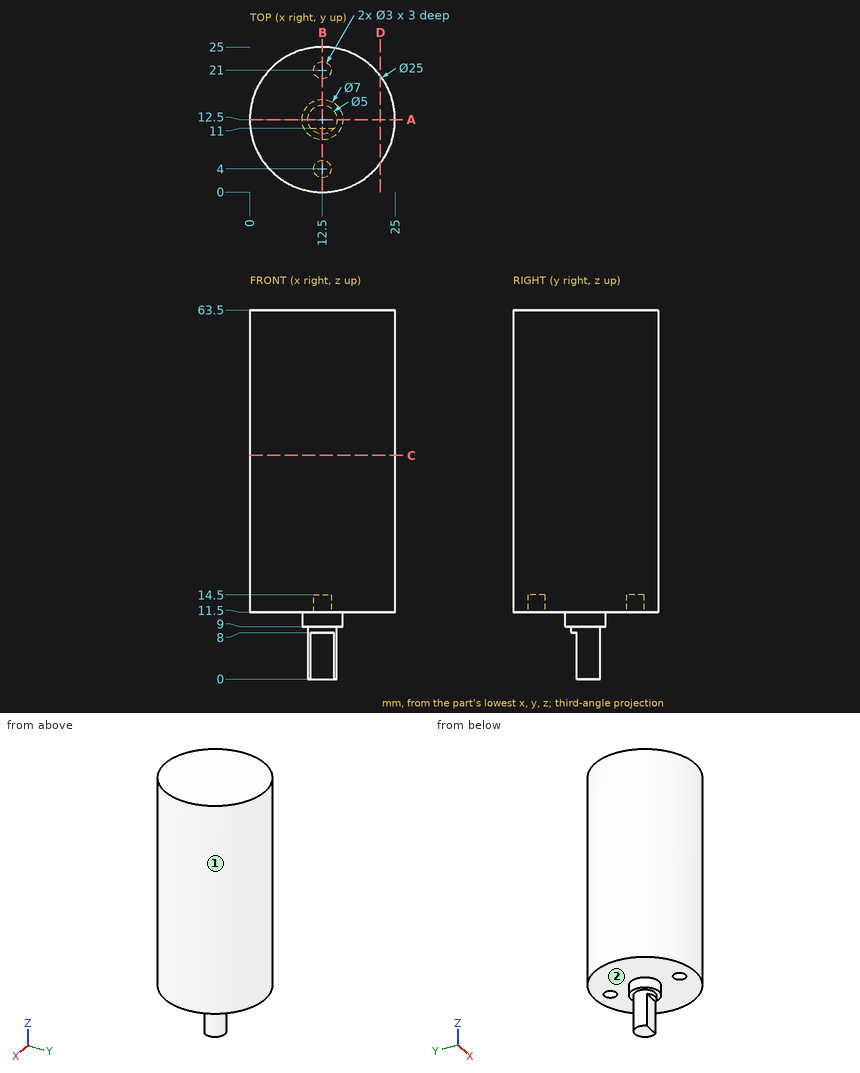
Drawing for the job (mm, zero at the part's lowest x, y, z). A direction names the side the tool comes from. Round coordinates to 2 decimals unless told otherwise and drop trailing zeros. Loops run counter-clockwise (first coordinate to the right, second up) from the corner with the lowest first, then second, coordinate; pieces in that order, holes last.
1. Drop flat-ended pins along their axis: P1, Ø12, axis at x = 4.5, z = 7.5, coming from the +Y side; P2, Ø6, axis at x = 8.5, z = 52.5, coming from the +Y side; P3, Ø6, axis at x = 19.5, z = 43.5, coming from the -Y side; P4, Ø5.5, axis at x = 11, y = 11.5, coming from the -Z side. Give the stop position or say it passes through.
Check values:
P1: stops at y = 24.49
P2: stops at y = 24.96
P3: stops at y = 0.66
P4: stops at z = 0
2. Band-saw the part on A-A, the plane y = 12.5. List the corners of the cut face in (x, z), and give its area (3 significant figures).
Check values:
outline: (0, 11.5) - (9, 11.5) - (9, 9) - (10, 9) - (10, 0) - (15, 0) - (15, 9) - (16, 9) - (16, 11.5) - (25, 11.5) - (25, 63.5) - (0, 63.5) - close
area: 1,360 mm2
3. Tool access for the marked faces 1 and 2: list every direction of +Z, -Z, +X, -X, +Y, -Y with a clear straight run to the whole face (end or side of a thin tool).
Check values:
face 1: +Z, -Z
face 2: -Z
4. Wall check: probe 1 along Y at (x, z) = (12.5, 12.55); probe 2 along Z at (x, y) = (19, 12.25); probe 3 along Y at (x, z) = (13, 54). Give the ranges that are in metal, low to high.
Check values:
probe 1: y = 0 to 2.5, 5.5 to 19.5, 22.5 to 25
probe 2: z = 11.5 to 63.5
probe 3: y = 0.01 to 24.99
5. Band-saw the part on B-B, the plane x = 12.5. List the corners of the cut face in (y, z), and give its area (3 significant figures).
Check values:
outline: (0, 11.5) - (2.5, 11.5) - (2.5, 14.5) - (5.5, 14.5) - (5.5, 11.5) - (9, 11.5) - (9, 9) - (10, 9) - (10, 8) - (11, 8) - (11, 0) - (15, 0) - (15, 9) - (16, 9) - (16, 11.5) - (19.5, 11.5) - (19.5, 14.5) - (22.5, 14.5) - (22.5, 11.5) - (25, 11.5) - (25, 63.5) - (0, 63.5) - close
area: 1,340 mm2
6. Band-saw the part on C-C, the plane z = 38.5. List the corners of the cut face in (x, y), and give its area (3 significant figures).
Check values:
outline: circle Ø25 at (12.5, 12.5)
area: 491 mm2
7. Band-saw the part on D-D, the plane x = 22.5. List the corners of the cut face in (y, z), and give its area (3 significant figures).
Check values:
outline: (5, 11.5) - (20, 11.5) - (20, 63.5) - (5, 63.5) - close
area: 780 mm2
